Verification items for the finished model (mm, model axes). A direction names the side the tool comes from. Give positions to 0.01 mm unless a question says otherwise; leave off trailing zeros. Write each loop counter-clockwise with the first axis right and the second up, starting at its lowest first coordinate (ties: lowest second). Pieces come first, ordered by that corner, then holes. Notation, with made-up numbers: (-2, 9) -> (13, 9) arc R7 ccw to (13, 21) -> close; hole circle Ø10 at (35.25, 57.5). An arc over 180 degrees is marked (long way). Answer as CSV lines item,"result".
Autodesk Inventor part; units mm, degrees
ref_plane "YZ Plane" through (0, 0, 0) normal (1, 0, 0) x (0, 1, 0)
ref_plane "XZ Plane" through (0, 0, 0) normal (0, 1, 0) x (-1, 0, 0)
ref_plane "XY Plane" through (0, 0, 0) normal (0, 0, 1) x (1, 0, 0)
sketch "Sketch1" plane through (0, 0, 0) normal (1, 0, 0) x (0, 1, 0)
  circle A0 centre (0, 0) radius 16.5
  dimension "d0" = 33
extrude "Extrusion1" add sketch "Sketch1" along normal blind 40.5
sketch "Sketch2" plane through (40.5, 0, 0) normal (1, 0, 0) x (0, 0, -1)
  circle A0 centre (0, 0) radius 16.5
  circle A1 centre (0, -5.5) radius 5
extrude "Extrusion2" add sketch "Sketch2" along normal blind 2.5 contours A1
sketch "Sketch3" plane through (43, -5.5, 0) normal (1, 0, 0) x (0, 0, -1)
  circle A0 centre (0, 0) radius 2.5
  point P0 (0, 5.5)
  dimension "d7" = 5
extrude "Extrusion3" add sketch "Sketch3" along normal blind 8.5
sketch "Sketch4" plane through (40.5, 0, 0) normal (1, 0, 0) x (0, 0, -1)
  circle A0 centre (0, 0) radius 16.5
  circle A1 centre (0, 13.5) radius 1.25
  circle A2 centre (-11.6913, -6.75) radius 1.25
  circle A3 centre (11.6913, -6.75) radius 1.25
  dimension "d11" = 2.5
  dimension "d14" = 360
extrude "Extrusion4" cut sketch "Sketch4" against normal blind 8.5 contours A1 | A2 | A3
properties part number "Motor"
1) Section check B-B (z = 0). Record the boundary of the cut face in (x, y), and give its area (3 significant figures).
Reported:
outline,"(0, -16.5) -> (40.5, -16.5) -> (40.5, -10.5) -> (43, -10.5) -> (43, -8) -> (51.5, -8) -> (51.5, -3) -> (43, -3) -> (43, -0.5) -> (40.5, -0.5) -> (40.5, 12.25) -> (32, 12.25) -> (32, 14.75) -> (40.5, 14.75) -> (40.5, 16.5) -> (0, 16.5) -> close"
area,"1,380 mm²"
2) Section check D-D (x = 10.5). Record the boundary of the cut face in (y, z), and give its area (3 significant figures).
Reported:
outline,"circle Ø33 at (0, 0)"
area,"855 mm²"
3) Scan lines: line 1 along X through (y, z) = (-1, 14); line 2 along Z through (x, y) = (36, -6); line 3 along Z through (x, y) = (26.5, -14). Record each from-to range of solid material in increasing order.
Reported:
line 1,"0 to 40.5"
line 2,"-15.37 to -12.69, -10.69 to 10.69, 12.69 to 15.37"
line 3,"-8.73 to 8.73"
4) Depth check by flat-ended pin: pin 1 (1.5 mm diameter, centred on y = 13.5, z = 0, fed in from +X); pin 2 (1 mm diameter, centred on x = 15.5, y = 8.5, fed in from +Z); pin 3 (6 mm diameter, centred on x = 22, y = -9.5, fed in from +Z); pin 4 (8 mm diameter, centred on x = 17.5, z = -1.5, fed in from +Y). Enter the tip coordinate at first touch or a pass-through.
Reported:
pin 1,"x = 32"
pin 2,"z = 14.43"
pin 3,"z = 15.17"
pin 4,"y = 16.5"
5) Tool access check on faces 4 (the cylindrical face through (41.73, -0.62, 1.08)), 5 (the flat face through (0, 0, 0)). Record the directions out of +Z, -Z, +X, -X, +Y, -Y that give a thin tool (end or side, any length) a straight path to the whole face; none if there is none.
Reported:
face 4,"+X"
face 5,"+Z, -Z, -X, +Y, -Y"
6) Section check A-A (x = 36.5). Record the boundary of the cut face in (y, z).
Reported:
outline,"circle Ø33 at (0, 0); hole circle Ø2.5 at (-6.75, -11.69); hole circle Ø2.5 at (-6.75, 11.69); hole circle Ø2.5 at (13.5, 0)"
7) Section check C-C (y = -1.5). Record the boundary of the cut face in (x, z), and give its area (3 significant figures).
Reported:
outline,"(0, -16.43) -> (40.5, -16.43) -> (40.5, -3) -> (43, -3) -> (43, 3) -> (40.5, 3) -> (40.5, 16.43) -> (0, 16.43) -> close"
area,"1,350 mm²"
8) Draft check along Z on faces 1 (the cylindrical face through (36.31, -7.229, 10.537)), 2 (the cylindrical face through (19.97, 15.24, 6.32)), 3 (the flat face through (43, -3, -1)). Enter one of: +Z half, -Z half, draft (parallel to the pull), parting line (faces both ways), or undercut.
Reported:
face 1,"undercut"
face 2,"parting line"
face 3,"draft"
